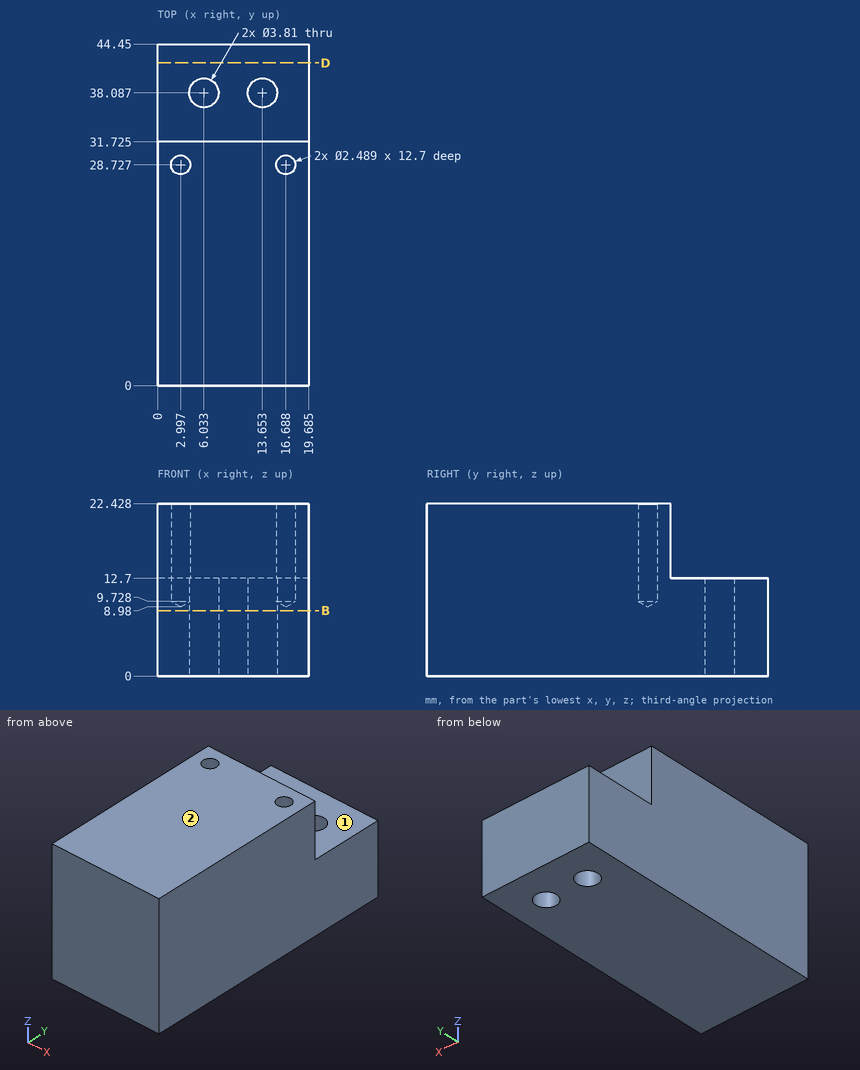
Here's the drawing with two shaded views (mm, measured from the low corner). I have some questions. A direction names the side the tool comes from. Coordinates: 2 decimals unless noted, no trailing zeros. Order: outer loops, then holes, each group sorted by start corner. A loop starts at its lowest first (then second) coordinate and runs counter-clockwise, first axis right, second up.
Item 1: I'm going to push flat-ended pins straight in: pin 1 Ø2 at (x, y) = (16, 35) entering from -Z; pin 2 Ø2 at (x, y) = (16.69, 28.73) entering from +Z; pin 3 Ø8 at (x, z) = (14.5, 19) entering from +Y (1 decimal); pin 4 Ø8 at (y, z) = (37, 19.5) entering from +X. Where does each tip first touch, or does it pass through?
Response values:
pin 1: stops at z = 0
pin 2: stops at z = 9.58
pin 3: stops at y = 31.7
pin 4: passes through
Item 2: Which directions (+Z, -Z, +X, -X, +Y, -Y) give clear straight access to the entire face, cutting with the end or side of a thin tool? Please do the marked faces 1 and 2.
Response values:
face 1: +Z, +X, -X, +Y
face 2: +Z, +X, -X, +Y, -Y
Item 3: If we section it at D-D, the plane y = 42: List the corners of the cut face in (x, z) for me (1 decimal), then the cut area to 3 significant figures.
Response values:
outline: (0, 0) - (19.7, 0) - (19.7, 12.7) - (0, 12.7) - close
area: 250 mm2
Item 4: I need wall thicknesses on probe 1 along Y at (x, z) = (6, 9.5); probe 2 along Y at (x, z) = (16, 16) (1 decimal); probe 3 along Z at (x, y) = (16, 36.5). Which ranges of each line are inside material? Lowest first, please.
Response values:
probe 1: y = 0 to 36.18, 39.99 to 44.45
probe 2: y = 0 to 27.7, 29.8 to 31.7
probe 3: z = 0 to 12.7
Item 5: If we section it at B-B, the plane z = 8.5: Give the number of separate pieces and of enclosed holes in the cut face, then the cut area to 3 significant figures.
Response values:
separate pieces: 1
enclosed holes: 2
area: 852 mm2
